from build123d import *

# Parameters (mm, degrees)
SKETCH1_R           = 38.1
SKETCH1_R_2         = 2.54
BOSS_EXTRUDE1_DEPTH = 12.7
SKETCH2_R           = 4
CUT_EXTRUDE1_DEPTH  = 56.358016583
SKETCH3_R           = 9.525
CUT_EXTRUDE2_DEPTH  = 6.35
SKETCH4_R           = 4
CUT_EXTRUDE3_DEPTH  = 56.358016583
SKETCH5_R           = 9.525
CUT_EXTRUDE5_DEPTH  = 6.35


with BuildPart() as part:
    # Sketch1 → Boss-Extrude1 (new body)
    with BuildSketch(Plane.XY):
        Circle(SKETCH1_R)
        with Locations((12, 0)):
            Circle(SKETCH1_R_2, mode=Mode.SUBTRACT)
        with Locations((0, -12)):
            Circle(SKETCH1_R_2, mode=Mode.SUBTRACT)
        with Locations((-12, 0)):
            Circle(SKETCH1_R_2, mode=Mode.SUBTRACT)
        with Locations((0, 12)):
            Circle(SKETCH1_R_2, mode=Mode.SUBTRACT)
    extrude(amount=BOSS_EXTRUDE1_DEPTH)

    # Sketch2 → Cut-Extrude1 (cut, through all)
    with BuildSketch(Plane.XY):
        with Locations((19.05, -19.05)):
            Circle(SKETCH2_R)
    extrude(amount=CUT_EXTRUDE1_DEPTH, mode=Mode.SUBTRACT)

    # Sketch3 → Cut-Extrude2 (cut)
    with BuildSketch(Plane.XY):
        with Locations((19.05, -19.05)):
            Circle(SKETCH3_R)
    extrude(amount=CUT_EXTRUDE2_DEPTH, mode=Mode.SUBTRACT)

    # Sketch4 → Cut-Extrude3 (cut, through all)
    with BuildSketch(Plane.XY):
        with Locations((-19.05, 19.05)):
            Circle(SKETCH4_R)
    extrude(amount=CUT_EXTRUDE3_DEPTH, mode=Mode.SUBTRACT)

    # Sketch5 → Cut-Extrude5 (cut)
    with BuildSketch(Plane.XY):
        with Locations((-19.05, 19.05)):
            Circle(SKETCH5_R)
    extrude(amount=CUT_EXTRUDE5_DEPTH, mode=Mode.SUBTRACT)


solid = part.part
Work out the finished part from the listing and answer in its coordinate system (mm). A direction names the side the tool comes from. Round coordinates to 2 decimals unless told otherwise and drop trailing zeros. Write each loop counter-clockwise with the first axis right and the second up, starting at its lowest first coordinate (ties: lowest second). Pieces come first, ordered by that corner, then holes. Notation, with made-up numbers: M 38,-39 L 42,-39 A6 cw 42,-35 Z; hole C -22.75,60.25 d11. An arc over 180 degrees is marked long. Use a Markdown table: item, result.
1) Determine the mould class of faces 1 (the face through (-15, 17, 6.35)), 2 (the face through (-30.235, -23.183, 6.261)), 3 (the face through (-1, 1, 0)) for opening direction X: pulls with the +X half, pulls with the -X half, needs draft (parallel to the pull), parting line crosses it, or undercut.
Taken from the geometry:
| item | result |
|---|---|
| face 1 | undercut |
| face 2 | parting line crosses it |
| face 3 | needs draft |
2) The part is cut by section A-A on y = 0. Give the vertices of the cut face in (x, z).
Taken from the geometry:
| item | result |
|---|---|
| outline | M -38.1,0 L -14.54,0 L -14.54,12.7 L -38.1,12.7 Z; M -9.46,0 L 9.46,0 L 9.46,12.7 L -9.46,12.7 Z; M 14.54,0 L 38.1,0 L 38.1,12.7 L 14.54,12.7 Z |
3) Flat-ended cylindrical pins translate along their axes: pin 1 (4 mm diameter, centred on y = -4.5, z = 11, fed in from -X); pin 2 (1.5 mm diameter, centred on x = -15.5, z = 3.5, fed in from -Y); pin 3 (1.5 mm diameter, centred on x = 27.5, z = 2.5, fed in from +Y). Find the tip coordinate at first contact, or state that the pin passes through.
Taken from the geometry:
| item | result |
|---|---|
| pin 1 | stops at x = -38.02 |
| pin 2 | stops at y = -35.13 |
| pin 3 | stops at y = 27.13 |
4) The part is cut by section D-D on y = 19.05. Give the vertices of the cut face in (x, z) (3 decimals), plus the area to 3 significant figures.
Taken from the geometry:
| item | result |
|---|---|
| outline | M -32.996,0 L -28.575,0 L -28.575,6.35 L -23.05,6.35 L -23.05,12.7 L -32.996,12.7 Z; M -15.05,6.35 L -9.525,6.35 L -9.525,0 L 32.996,0 L 32.996,12.7 L -15.05,12.7 Z |
| area | 666 mm2 |
5) The part is cut by section C-C on z = 11.75. Give the vertices of the cut face in (x, y), plus the area to 3 significant figures.
Taken from the geometry:
| item | result |
|---|---|
| outline | C 0,0 d76.2; hole C -19.05,19.05 d8; hole C -12,0 d5.08; hole C 0,-12 d5.08; hole C 0,12 d5.08; hole C 12,0 d5.08; hole C 19.05,-19.05 d8 |
| area | 4,380 mm2 |
6) Consider line 1 (Y direction, x = 0, z = 3.25); line 2 (Y direction, x = -12, z = 3.25); line 3 (Y direction, x = -19, z = 11.25). Determine where each line is inside the solid, lowest interval first. Write a range as [from, to].
Taken from the geometry:
| item | result |
|---|---|
| line 1 | y = [-38.1, -14.54], [-9.46, 9.46], [14.54, 38.1] |
| line 2 | y = [-36.16, -2.54], [2.54, 12.65], [25.45, 36.16] |
| line 3 | y = [-33.02, 15.05], [23.05, 33.02] |
7) Which of the six approach directions +Z, -Z, +X, -X, +Y, -Y give full straight-line access (tool end or side, diameter ignored) to faces 4 (the face through (17.81, -9.606, 3.131)), 5 (the face through (-1, 1, 12.7))?
Taken from the geometry:
| item | result |
|---|---|
| face 4 | -Z |
| face 5 | +Z, +X, -X, +Y, -Y |
